Source: three-view drawing plus pictorial views. Frame: mm from the lowest corner of the part. A direction names the side the tool comes from. Give positions to 0.01 mm unless a question says otherwise; leave off trailing zeros. Write each loop counter-clockwise with the first axis right and the second up, starting at its lowest first coordinate (ties: lowest second). Pieces come first, ordered by that corner, then holes. Notation, with made-up numbers: (37, 27.5) -> (73, 27.5) arc R11 cw to (73, 45.5) -> close; hole circle Ø2 at (15.25, 15.5). An arc over 180 degrees is marked (long way). Answer in a Markdown table with one row per item. Add a question column.
Item 1: Access query for the marked faces 1 and 2. Directions: +Z, -Z, +X, -X, +Y, -Y. A direction counts if a zero-diameter tool reaches every point of the face in a straight line with its end or side. Return the directions, or none.
Item 2: Section query A-A on y = 3. Output: boundary loops of the cut face in (x, z), plus the area to 3 significant figures.
Item 3: Section query B-B on x = 2. Output: boundary loops of the cut face in (y, z).
Item 4: First-contact query: P1, Ø6, axis at x = 10.5, z = 10.5, coming from the +Y side; P2, Ø1, axis at y = 1, z = 7, coming from the -X side; P3, Ø0.6, axis at y = 0.5, z = 11.5, coming from the +X side. Flat tips, straight axial feed; report the tip coordinate or a pass-through.
Item 5: Section query C-C on x = 8.5. Output: boundary loops of the cut face in (y, z).
Item 6: Material intervals for probe 1 along Z at (x, y) = (1.75, 8); probe 2 along Y at (x, z) = (10.5, 12.5), sorted ascending. Write a range as from..to.
Item 7: Section query D-D on z = 17.75. Output: boundary loops of the cut face in (x, y).
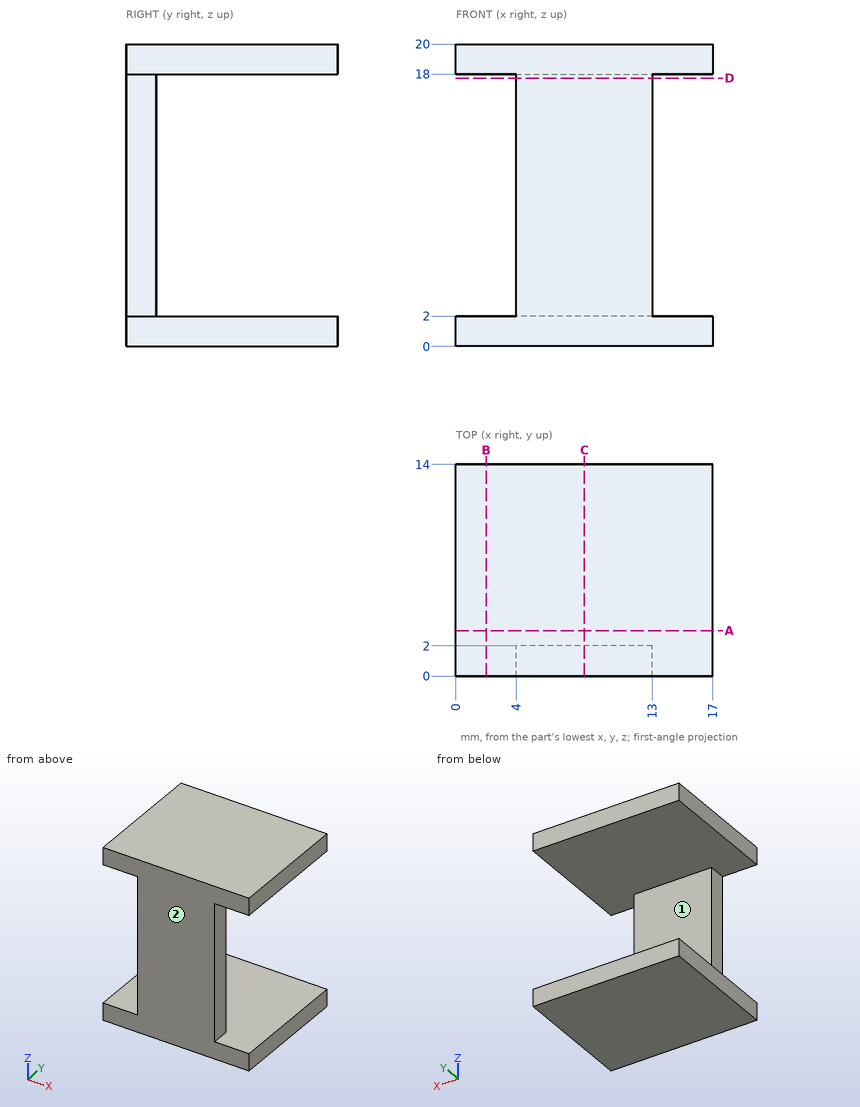
Findings below:
| question | item | result |
|---|---|---|
| 1 | face 1 | +X, -X, +Y |
| 1 | face 2 | +Z, -Z, +X, -X, -Y |
| 2 | outline | (0, 0) -> (17, 0) -> (17, 2) -> (0, 2) -> close; (0, 18) -> (17, 18) -> (17, 20) -> (0, 20) -> close |
| 2 | area | 68.0 mm^2 |
| 3 | outline | (0, 0) -> (14, 0) -> (14, 2) -> (0, 2) -> close; (0, 18) -> (14, 18) -> (14, 20) -> (0, 20) -> close |
| 4 | P1 | stops at y = 2 |
| 4 | P2 | stops at x = 4 |
| 4 | P3 | stops at x = 13 |
| 5 | outline | (0, 0) -> (14, 0) -> (14, 2) -> (2, 2) -> (2, 18) -> (14, 18) -> (14, 20) -> (0, 20) -> close |
| 6 | probe 1 | z = 0..2, 18..20 |
| 6 | probe 2 | y = 0..2 |
| 7 | outline | (4, 0) -> (13, 0) -> (13, 2) -> (4, 2) -> close |
